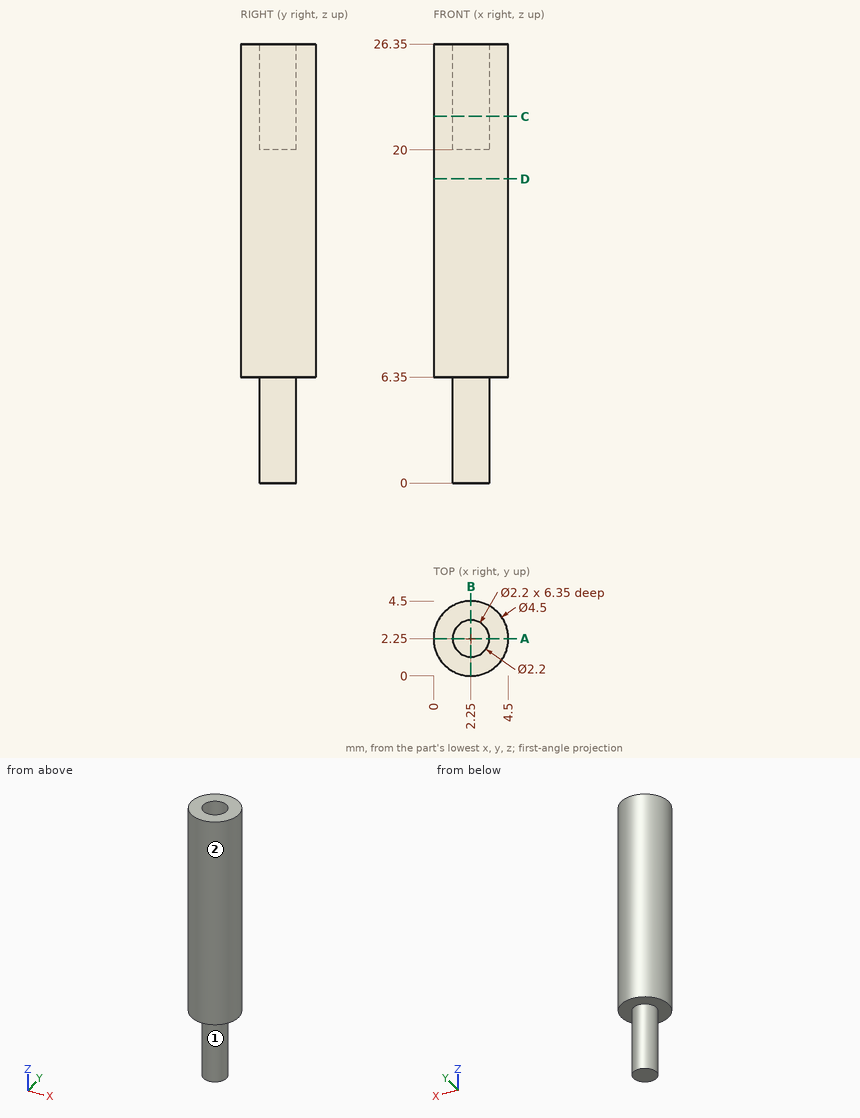
Design review of the part shown in the three views and the two pictorial views. Dimensions are in mm from the part's minimum x, y and z. A direction names the side the tool comes from. Coordinates: 2 decimals unless noted, no trailing zeros. Write each loop counter-clockwise with the first axis right and the second up, starting at its lowest first coordinate (ties: lowest second). Pieces come first, ordered by that corner, then holes. Notation, with made-up numbers: (75, 59) -> (109, 59) arc R22 ccw to (109, 98) -> close; hole circle Ø5 at (-36.75, 72.25). An arc over 180 degrees is marked (long way). Answer in a Markdown table with one row per item.
1. We need section A-A, the plane y = 2.25. State the section outline as (x, z) points.
Answers below:
| item | result |
|---|---|
| outline | (0, 6.35) -> (1.15, 6.35) -> (1.15, 0) -> (3.35, 0) -> (3.35, 6.35) -> (4.5, 6.35) -> (4.5, 26.35) -> (3.35, 26.35) -> (3.35, 20) -> (1.15, 20) -> (1.15, 26.35) -> (0, 26.35) -> close |
2. We need section D-D, the plane z = 18.25. State the section outline as (x, y) points, and give its area (3 significant figures).
Answers below:
| item | result |
|---|---|
| outline | circle Ø4.5 at (2.25, 2.25) |
| area | 15.9 mm^2 |
3. Wall thickness on probe 1 along Y at (x, z) = (2.25, 23); probe 2 along Z at (x, y) = (1, 3.85); probe 3 along Z at (x, y) = (1.2, 2.1): over which ranges is each line inside the solid? List them lowest first. Write a range as [from, to].
Answers below:
| item | result |
|---|---|
| probe 1 | y = [0, 1.15], [3.35, 4.5] |
| probe 2 | z = [6.35, 26.35] |
| probe 3 | z = [0, 20] |
4. We need section C-C, the plane z = 22. State the section outline as (x, y) points, and give its area (3 significant figures).
Answers below:
| item | result |
|---|---|
| outline | circle Ø4.5 at (2.25, 2.25); hole circle Ø2.2 at (2.25, 2.25) |
| area | 12.1 mm^2 |
5. Clearance check with a flat-ended pin moving along its axis: pin 1 Ø1.5 at (y, z) = (2.5, 21.5) entering from -X. State where the tip first meets the part, or that it passes through.
Answers below:
| item | result |
|---|---|
| pin 1 | stops at x = 0 |
6. For the marked faces 1 and 2, list the 3-axis set-ups (+Z, -Z, +X, -X, +Y, -Y) from which the entire face can be reached by the end or side of a thin tool; tool diameter is ignored.
Answers below:
| item | result |
|---|---|
| face 1 | -Z |
| face 2 | +Z, -Z |
